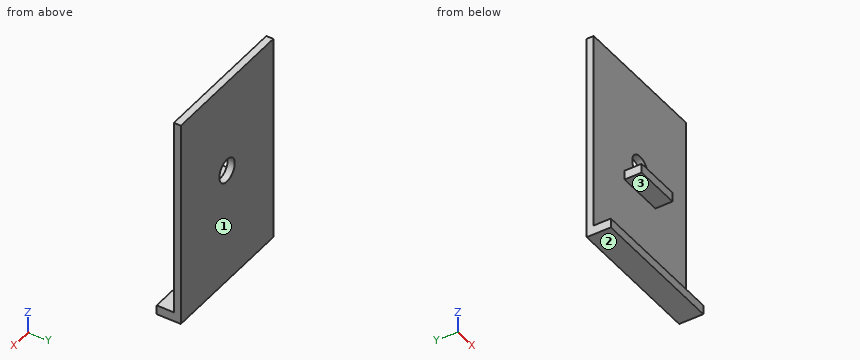
from build123d import *

# Parameters (mm, degrees)
F0_W     = 60
F0_H     = 90
F2_DEPTH = 3
F1_R     = 5
F3_DEPTH = 25.4
F4_W     = 60
F4_H     = 10.3
F5_DEPTH = 4
F6_W     = 20
F6_H     = 4
F7_DEPTH = 10.3


with BuildPart() as f2:
    # F0 (on Front) → F2 (new body)
    with BuildSketch(Plane.XZ):
        with Locations((0, -5)):
            Rectangle(F0_W, F0_H)
    extrude(amount=F2_DEPTH)

    # F1 (on face) → F3 (cut)
    with BuildSketch(Plane.XZ):
        Circle(F1_R)
    extrude(amount=F3_DEPTH, mode=Mode.SUBTRACT)

    # F4 (on face) → F5 (join)
    with BuildSketch(Plane(origin=(0, 0, -50), x_dir=(1, 0, 0), z_dir=(0, 0, -1))):
        with Locations((0, 5.15)):
            Rectangle(F4_W, F4_H)
    extrude(amount=-F5_DEPTH)

    # F6 (on Front) → F7 (join)
    with BuildSketch(Plane.XZ):
        with Locations((0, -10)):
            Rectangle(F6_W, F6_H)
    extrude(amount=F7_DEPTH)


solid = f2.part
Input: part model. Units: mm. Frame: model coordinates. Face numbers are marked on the shaded views. Coordinates: 2 decimals unless noted, no trailing zeros. Order: outer loops, then holes, each group sorted by start corner. A loop starts at its lowest first (then second) coordinate and runs counter-clockwise, first axis right, second up. Notation, with made-up numbers: M 32,10 L 61,10 A22 ccw 61,48 Z; hole C 45,-22 d7. An arc over 180 degrees is marked long. Answer in a Markdown table with one row per item.
(1) Section query C-C, the plane z = -2. Output: boundary loops of the cut face in (x, y), plus the area to 3 significant figures.
Numbers:
| item | result |
|---|---|
| outline | M -30,-3 L -4.58,-3 L -4.58,0 L -30,0 Z; M 4.58,-3 L 30,-3 L 30,0 L 4.58,0 Z |
| area | 153 mm^2 |
(2) Draft query along Z for the marked faces 1, 2 and 3. Return one class per face: pulls with the +Z half, pulls with the -Z half, needs draft (parallel to the pull), parting line crosses it, or undercut.
Numbers:
| item | result |
|---|---|
| face 1 | needs draft |
| face 2 | pulls with the -Z half |
| face 3 | undercut |
(3) Material intervals for line 1 (Z direction, x = 0, y = -2.15); line 2 (Z direction, x = -9.5, y = -9.25); line 3 (X direction, y = -1.3, z = 0), sorted ascending. Write a range as [from, to].
Numbers:
| item | result |
|---|---|
| line 1 | z = [-50, -5], [5, 40] |
| line 2 | z = [-50, -46], [-12, -8] |
| line 3 | x = [-30, -5], [5, 30] |
(4) Section query A-A, the plane x = 3. Output: boundary loops of the cut face in (y, z).
Numbers:
| item | result |
|---|---|
| outline | M -10.3,-50 L 0,-50 L 0,-4 L -3,-4 L -3,-8 L -10.3,-8 L -10.3,-12 L -3,-12 L -3,-46 L -10.3,-46 Z; M -3,4 L 0,4 L 0,40 L -3,40 Z |
(5) Contact query for flat-ended pins moving along their axis: pin 1 Ø2 at (y, z) = (-7, -10) entering from +X; pin 2 Ø8 at (x, z) = (0, 0) entering from +Y; pin 3 Ø2 at (x, y) = (4, -6) entering from +Z; pin 4 Ø18 at (x, z) = (10.5, 6) entering from -Y. Output: stop coordinate, or through.
Numbers:
| item | result |
|---|---|
| pin 1 | stops at x = 10 |
| pin 2 | passes through |
| pin 3 | stops at z = -8 |
| pin 4 | stops at y = -3 |
(6) Section query D-D, the plane x = -9. Output: boundary loops of the cut face in (y, z).
Numbers:
| item | result |
|---|---|
| outline | M -10.3,-50 L 0,-50 L 0,40 L -3,40 L -3,-8 L -10.3,-8 L -10.3,-12 L -3,-12 L -3,-46 L -10.3,-46 Z |
(7) Section query B-B, the plane y = -6. Output: boundary loops of the cut face in (x, z), plus the area to 3 significant figures.
Numbers:
| item | result |
|---|---|
| outline | M -30,-50 L 30,-50 L 30,-46 L -30,-46 Z; M -10,-12 L 10,-12 L 10,-8 L -10,-8 Z |
| area | 320 mm^2 |
